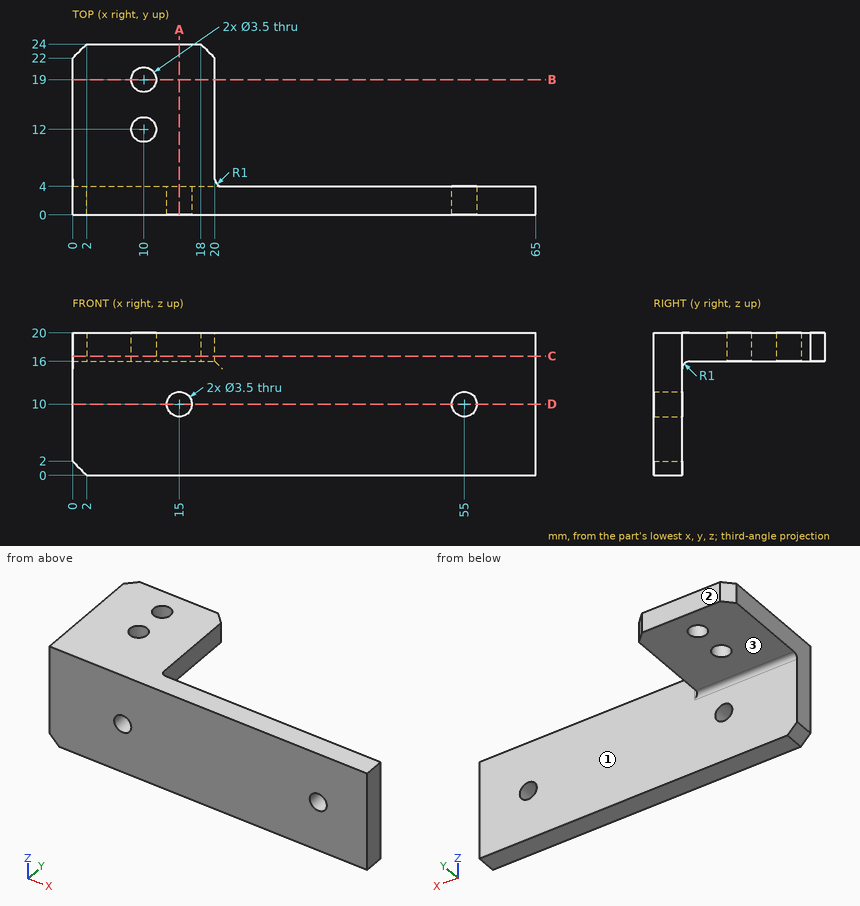
Job drawing, mm, ordinate dimensions from the low corner. One solid piece. A direction names the side the tool comes from. Give positions to 0.01 mm unless a question says otherwise; leave off trailing zeros. Order: outer loops, then holes, each group sorted by start corner. A loop starts at its lowest first (then second) coordinate and runs counter-clockwise, first axis right, second up. Notation, with made-up numbers: (-15.5, -23) - (14.5, -23) arc R20 ccw to (14.5, 1) - close; hole circle Ø1 at (80.5, 8). An arc over 180 degrees is marked (long way). Answer in a Markdown table with one row per item.
1. Saw through at B-B, the plane y = 19. Give the cut face in (x, z), plus the area to 3 significant figures.
Data:
| item | result |
|---|---|
| outline | (0, 16) - (8.25, 16) - (8.25, 20) - (0, 20) - close; (11.75, 16) - (20, 16) - (20, 20) - (11.75, 20) - close |
| area | 66.0 mm² |
2. Saw through at A-A, the plane x = 15. Give the cut face in (y, z), plus the area to 3 significant figures.
Data:
| item | result |
|---|---|
| outline | (0, 0) - (4, 0) - (4, 8.25) - (0, 8.25) - close; (0, 11.75) - (4, 11.75) - (4, 15) arc R1 cw to (5, 16) - (24, 16) - (24, 20) - (0, 20) - close |
| area | 146 mm² |
3. Probe probe 1 along Y at (x, z) = (10, 18.05); probe 2 along X at (y, z) = (1.75, 10); probe 3 along Z at (x, y) = (15, 1.7). List the from-to ranges inside material, lowest first. Write a range as [from, to].
Data:
| item | result |
|---|---|
| probe 1 | y = [0, 10.25], [13.75, 17.25], [20.75, 24] |
| probe 2 | x = [0, 13.25], [16.75, 53.25], [56.75, 65] |
| probe 3 | z = [0, 8.25], [11.75, 20] |
4. Flat gauge pins, fed straight in: pin 1 (6 mm diameter, centred on x = 22, z = 3.5, fed in from +Y); pin 2 (4 mm diameter, centred on y = 19, z = 12.5, fed in from -X); pin 3 (5.5 mm diameter, centred on x = 14.5, y = 17.5, fed in from -Z); pin 4 (10 mm diameter, centred on y = 15, z = 16, fed in from +X). Where does each tip first touch, or does it go through?
Data:
| item | result |
|---|---|
| pin 1 | stops at y = 4 |
| pin 2 | passes through |
| pin 3 | stops at z = 16 |
| pin 4 | stops at x = 20 |
5. Tool access for the marked faces 1, 2 and 3: list every direction of +Z, -Z, +X, -X, +Y, -Y with a clear straight run to the whole face (end or side of a thin tool).
Data:
| item | result |
|---|---|
| face 1 | -Z, +X, +Y |
| face 2 | +Z, -Z, +X, -X, +Y |
| face 3 | -Z, +X, -X, +Y |
6. Saw through at C-C, the plane z = 16.75. Give the cut face in (x, y), plus the area to 3 significant figures.
Data:
| item | result |
|---|---|
| outline | (0, 0) - (65, 0) - (65, 4) - (21, 4) arc R1 cw to (20, 5) - (20, 22) - (18, 24) - (2, 24) - (0, 22) - close; hole circle Ø3.5 at (10, 12); hole circle Ø3.5 at (10, 19) |
| area | 637 mm² |
7. Saw through at D-D, the plane z = 10. Give the cut face in (x, y), plus the area to 3 significant figures.
Data:
| item | result |
|---|---|
| outline | (0, 0) - (13.25, 0) - (13.25, 4) - (0, 4) - close; (16.75, 0) - (53.25, 0) - (53.25, 4) - (16.75, 4) - close; (56.75, 0) - (65, 0) - (65, 4) - (56.75, 4) - close |
| area | 232 mm² |
